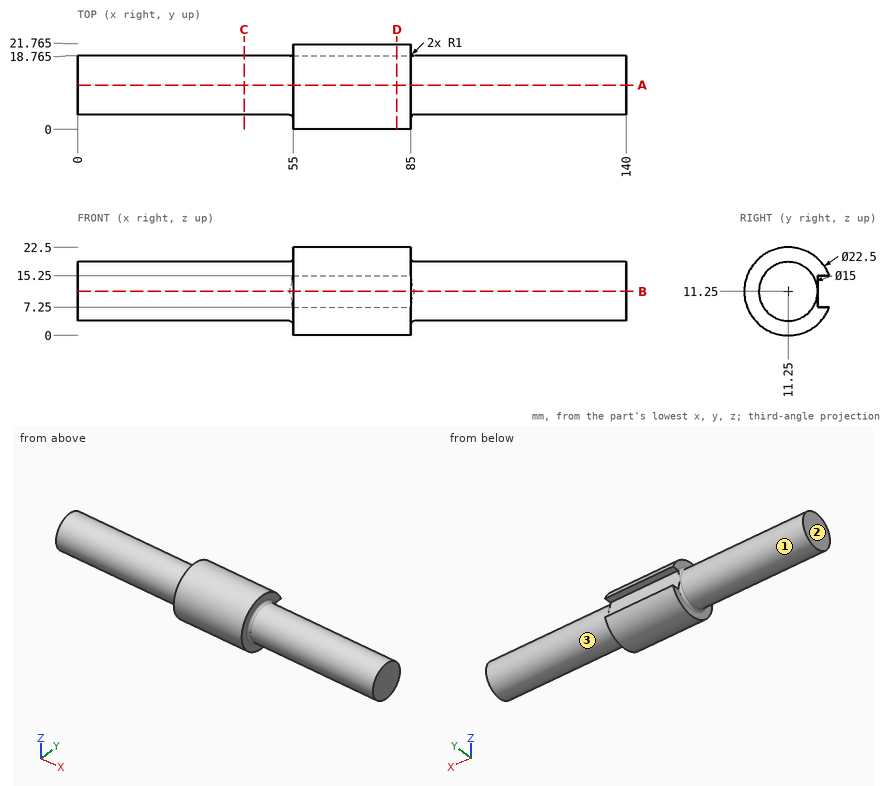
For this review, use the dimensioned drawing (mm, ordinates from the lowest corner) and the shaded views. A direction names the side the tool comes from. Round coordinates to 2 decimals unless told otherwise and drop trailing zeros. Write each loop counter-clockwise with the first axis right and the second up, starting at its lowest first coordinate (ties: lowest second). Pieces come first, ordered by that corner, then holes. Notation, with made-up numbers: (71, 49) -> (81, 49) arc R18 ccw to (81, 69) -> close; hole circle Ø6 at (45.5, 74). An arc over 180 degrees is marked (long way). Use one line per item in the form item = value.
Q1. Consider section C-C (x = 42.5). State the section outline as (y, z) points.
Resolved:
outline = circle Ø15 at (11.25, 11.25)
Q2. Consider section D-D (x = 81.5). State the section outline as (y, z) points (3 decimals), then the cut area to 3 significant figures.
Resolved:
outline = (18.765, 7.25) -> (18.765, 15.25) -> (21.765, 15.25) arc R11.25 ccw (long way) to (21.765, 7.25) -> close
area = 370 mm²
Q3. To check wall thickness, follow probe 1 along X at (y, z) = (18, 18.5); probe 2 along Z at (x, y) = (75, 12) (3 decimals); probe 3 along Y at (x, z) = (38, 8). State the ranges of each line that lie inside material, in increasing order. Write a range as from..to.
Resolved:
probe_1 = 55..85
probe_2 = 0.025..22.475
probe_3 = 4.49..18.01
Q4. Consider section B-B (z = 11.25). State the section outline as (x, y) points (3 decimals), then the cut area to 3 significant figures.
Resolved:
outline = (0, 3.75) -> (54, 3.75) arc R1 cw to (55, 2.75) -> (55, 0) -> (85, 0) -> (85, 2.75) arc R1 cw to (86, 3.75) -> (140, 3.75) -> (140, 18.75) -> (86, 18.75) arc R1 cw to (85.828, 18.765) -> (54.172, 18.765) arc R1 cw to (54, 18.75) -> (0, 18.75) -> close
area = 2,210 mm²
Q5. Clearance check with flat-ended pins moving along their axes: pin 1 Ø1.5 at (x, y) = (65, 20) entering from -Z; pin 2 Ø2 at (x, y) = (72, 8.5) entering from +Z; pin 3 Ø12 at (x, y) = (114, 11.5) entering from -Z. State where each tip first meets the part, or that it passes through.
Resolved:
pin_1 = 3.34
pin_2 = 22.36
pin_3 = 3.75
Q6. Machinability: for the marked faces 1, 2 and 3, which of the approach directions +Z, -Z, +X, -X, +Y, -Y give a long, thin tool a straight path to every point of the face, cutting with its end or side? Answer none if there is none.
Resolved:
face_1 = -X
face_2 = +Z, -Z, -X, +Y, -Y
face_3 = +X
Q7. Consider section A-A (y = 11.25). State the section outline as (x, z) points, then the cut area to 3 significant figures.
Resolved:
outline = (0, 3.75) -> (54, 3.75) arc R1 cw to (55, 2.75) -> (55, 0) -> (85, 0) -> (85, 2.75) arc R1 cw to (86, 3.75) -> (140, 3.75) -> (140, 18.75) -> (86, 18.75) arc R1 cw to (85, 19.75) -> (85, 22.5) -> (55, 22.5) -> (55, 19.75) arc R1 cw to (54, 18.75) -> (0, 18.75) -> close
area = 2,330 mm²
